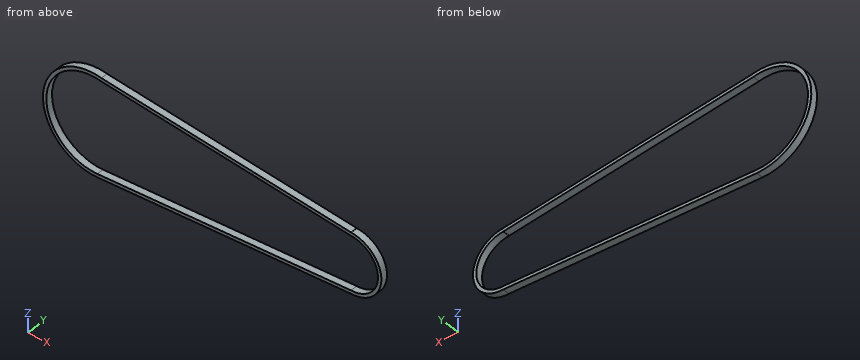
```python
from build123d import *

# Parameters (mm, degrees)
F1_DEPTH = 5


with BuildPart() as f1:
    # F0 (on Front) → F1 (new body, symmetric)
    with BuildSketch(Plane.XZ):
        with BuildLine():
            Line((0, 75), (11.6628740197, 74.0876330409))
            ThreePointArc((11.6628740197, 74.0876330409), (5.8492530264, 74.7715603624), (0, 75))
        make_face()
        with BuildLine():
            Line((381.7354142666, 45.1374825353), (11.6628740197, 74.0876330409))
            Line((11.6628740197, 74.0876330409), (0, 75))
            ThreePointArc((0, 75), (-74.9414408269, -2.9631818699), (5.9217365004, -74.7658547522))
            Line((5.9217365004, -74.7658547522), (381.7354142666, -45))
            ThreePointArc((381.7354142666, -45), (426.7354142666, 0), (381.7354142666, 45))
            Line((381.7354142666, 45), (381.7354142666, 45.1374825353))
        make_face()
        with BuildLine():
            ThreePointArc((5.5240677228, -69.7816929846), (-69.9454019537, -2.7641898524), (0, 70))
            ThreePointArc((0, 70), (5.4620559663, 69.7865742433), (10.8908049775, 69.1475984178))
            Line((10.8908049775, 69.1475984178), (381.7354142666, 40.1223305537))
            Line((381.7354142666, 40.1223305537), (381.7354142666, 40))
            ThreePointArc((381.7354142666, 40), (421.7354142666, 0), (381.7354142666, -40))
            Line((381.7354142666, -40), (5.5240677228, -69.7816929846))
        make_face(mode=Mode.SUBTRACT)
    extrude(amount=F1_DEPTH, both=True)


solid = f1.part
```
Part model, mm, in its own coordinate system. Give positions to 0.01 mm unless a question says otherwise; leave off trailing zeros. Write each loop counter-clockwise with the first axis right and the second up, starting at its lowest first coordinate (ties: lowest second). Pieces come first, ordered by that corner, then holes. Notation, with made-up numbers: (25, 14.5) -> (76, 14.5) arc R23 ccw to (76, 45.5) -> close; hole circle Ø11 at (-38.5, 43). An arc over 180 degrees is marked (long way). Put each result on its own line as item: value. Start each with the question number.
Item 1: Wall check: L1, parallel to X at y = 0, z = 0; L2, parallel to Z at x = 281, y = 2.75; L3, parallel to Z at x = 12, y = 1.5. Give the ranges that are in metal, low to high. Write a range as [from, to].
Item 2: Cut at C-C (z = 0). List the corners of the cut face in (x, y).
Item 3: Cut at A-A (x = 0). List the corners of the cut face in (y, z).
Item 4: Pin check, flat tips, straight feed: pin 1 Ø6 at (y, z) = (2.5, 33.5) entering from +X; pin 2 Ø2 at (x, y) = (128, -3.5) entering from -Z; pin 3 Ø1 at (y, z) = (-1.5, -12) entering from +X. Stop position of each tip, or through.
Item 5: Cut at B-B (y = -3). List the corners of the cut face in (x, z), then the cut area to 3 significant figures.
Answer list:
1. L1: x = [-75, -70], [421.74, 426.74]
1. L2: z = [-52.98, -47.97], [48.01, 53.02]
1. L3: z = [-74.28, -69.27], [69.06, 74.06]
2. outline: (-75, -5) -> (-70, -5) -> (-70, 5) -> (-75, 5) -> close; (421.74, -5) -> (426.74, -5) -> (426.74, 5) -> (421.74, 5) -> close
3. outline: (-5, -75) -> (5, -75) -> (5, -70) -> (-5, -70) -> close; (-5, 70) -> (5, 70) -> (5, 75) -> (-5, 75) -> close
4. pin 1: stops at x = 414.82
4. pin 2: stops at z = -65.18
4. pin 3: stops at x = 425.24
5. outline: (5.92, -74.77) -> (381.74, -45) arc R45 ccw to (381.74, 45) -> (381.74, 45.14) -> (11.66, 74.09) arc R75 ccw (long way) to start; hole (5.52, -69.78) -> (381.74, -40) arc R40 ccw to (381.74, 40) -> (381.74, 40.12) -> (10.89, 69.15) arc R70 ccw (long way) to start
5. area: 5,630 mm2
